Model file for the job. Use its own axes, mm. A direction names the side the tool comes from. Round coordinates to 2 decimals unless told otherwise and drop trailing zeros. Order: outer loops, then holes, each group sorted by start corner. A loop starts at its lowest first (then second) coordinate and runs counter-clockwise, first axis right, second up. Notation, with made-up numbers: (24.5, 89.25) - (30.5, 89.25) arc R10 ccw to (30.5, 105.25) - close; hole circle Ø10 at (-7.75, 25.5). An arc over 180 degrees is marked (long way). Put each result on its own line as item: value. Start each with the question number.
Item 1: Pin check, flat tips, straight feed: pin 1 Ø1.5 at (y, z) = (7.5, -4) entering from +X; pin 2 Ø2.5 at (y, z) = (3.5, -3) entering from -X; pin 3 Ø1 at (x, y) = (-4.5, 5) entering from +Z. Stop position of each tip, or through.
Item 2: Saw through at A-A on y = 5.5. List the corners of the cut face in (x, z), plus the area to 3 significant figures.
Item 3: Saw through at C-C on y = 2.25. List the corners of the cut face in (x, z).
Item 4: Saw through at B-B on z = -7.5. List the corners of the cut face in (x, y), plus the area to 3 significant figures.
Item 5: Saw through at D-D on z = -3.25. List the corners of the cut face in (x, y), plus the area to 3 significant figures.
Item 6: Mould opens along Y. For faces 3 (the face through (-1, 0, -11)), 4 (the face through (-1.862, 5, -5)), 5 (the face through (-7.1, 4.96, -4.78)) say: pulls with the +Y half, pulls with the -Y half, needs draft (parallel to the pull), parting line crosses it, or undercut.
Item 7: Which spindle directions (+Z, -Z, +X, -X, +Y, -Y) get a long thin tool onto all of the face, cutting with end or side? Do faces 1 (the face through (-5.862, 5, -5)), 2 (the face through (-0.67, 4.96, -4.78)). Say none if no direction does.
Item 8: Probe probe 1 along Y at (x, z) = (-1.5, -3.75); probe 2 along X at (y, z) = (5.5, -7.5); probe 3 along Z at (x, y) = (-6.5, 8). List the from-to ranges inside material, lowest first.
```python
from build123d import *

# Parameters (mm, degrees)
BOSS_EXTRUDE1_DEPTH     = 10
CUT_EXTRUDE1_DEPTH      = 10
CUT_EXTRUDE1_DEPTH_BACK = 10
SKETCH2_R               = 1


with BuildPart() as part:
    # Sketch1 → Boss-Extrude1 (new body)
    with BuildSketch(Plane(origin=(0, 0, 0), x_dir=(1, 0, 0), z_dir=(0, 1, 0))):
        with BuildLine():
            Line((-5.862008202, 2.231502929), (-5.862008202, 5.326619487))
            ThreePointArc((-5.862008202, 5.326619487), (-5.287227483, 10.80918754), (-0.612008202, 7.888357178))
            ThreePointArc((-0.612008202, 7.888357178), (-0.941177841, 6.463137897), (-1.862008202, 5.326619487))
            Line((-1.862008202, 5.326619487), (-1.862008202, 2.231502929))
            ThreePointArc((-1.862008202, 2.231502929), (1.036971284, 4.424255563), (2.137991798, 7.888357178))
            ThreePointArc((2.137991798, 7.888357178), (-7.326109817, 12.787336664), (-5.862008202, 2.231502929))
        make_face()
    extrude(amount=BOSS_EXTRUDE1_DEPTH)

    # Sketch2 → Cut-Extrude1 (cut, two sides: drawn at the far end of the back side and taken through both)
    with BuildSketch(Plane(origin=(-5.862008202, 0, 0), x_dir=(0, 0, -1), z_dir=(1, 0, 0)).offset(-CUT_EXTRUDE1_DEPTH_BACK)):
        with Locations(Location((3.779061208, 5, 0), (0, 0, 180))):
            Circle(SKETCH2_R)
    extrude(amount=CUT_EXTRUDE1_DEPTH + CUT_EXTRUDE1_DEPTH_BACK, mode=Mode.SUBTRACT)


solid = part.part
```
Results found:
1. pin 1: stops at x = 1.25
1. pin 2: stops at x = -8.63
1. pin 3: stops at z = -10.93
2. outline: (-8.91, -4.65) arc R6 ccw (long way) to (1.19, -4.65) - (-1.86, -4.65) - (-1.86, -5.33) arc R3.25 cw (long way) to (-5.86, -5.33) - (-5.86, -4.65) - close; (-7.22, -2.91) - (-5.86, -2.91) - (-5.86, -2.23) arc R6 ccw to start; (-1.86, -2.91) - (-0.51, -2.91) arc R6 ccw to (-1.86, -2.23) - close
2. area: 60.5 mm²
3. outline: (-5.86, -5.33) - (-5.86, -2.23) arc R6 ccw (long way) to (-1.86, -2.23) - (-1.86, -5.33) arc R3.25 cw (long way) to start
4. outline: (-9.85, 0) - (-7.09, 0) - (-7.09, 10) - (-9.85, 10) - close; (-0.64, 0) - (2.13, 0) - (2.13, 10) - (-0.64, 10) - close
4. area: 55.2 mm²
5. outline: (-7.67, 0) - (-5.86, 0) - (-5.86, 4.15) - (-7.67, 4.15) - close; (-7.67, 5.85) - (-5.86, 5.85) - (-5.86, 10) - (-7.67, 10) - close; (-1.86, 0) - (-0.06, 0) - (-0.06, 4.15) - (-1.86, 4.15) - close; (-1.86, 5.85) - (-0.06, 5.85) - (-0.06, 10) - (-1.86, 10) - close
5. area: 30.0 mm²
6. face 3: pulls with the -Y half
6. face 4: needs draft
6. face 5: undercut
7. face 1: +Z, +Y, -Y
7. face 2: +X, -X
8. probe 1: y = 0 to 4, 6 to 10
8. probe 2: x = -9.85 to -7.09, -0.64 to 2.13
8. probe 3: z = -13.28 to -9.79, -5.99 to -2.5
